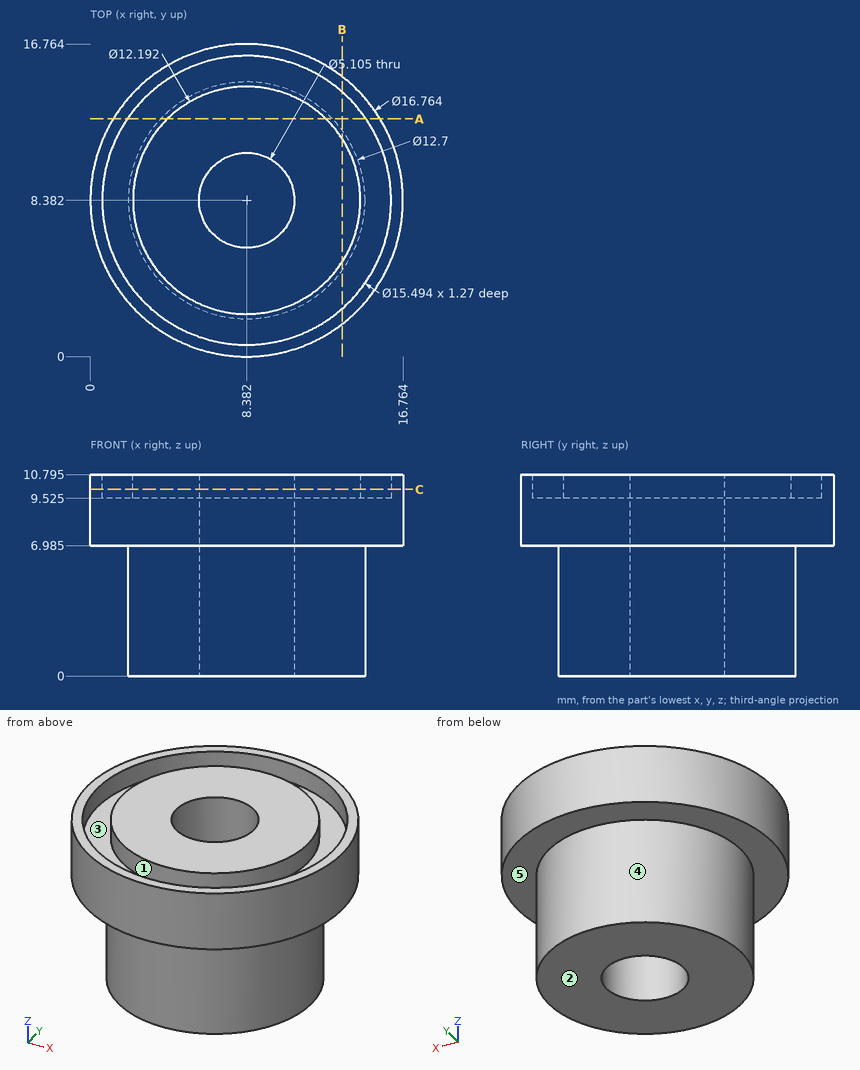
Part print with two shaded views. Sizes in mm from the minimum x, y, z corner. A direction names the side the tool comes from. Round coordinates to 2 decimals unless told otherwise and drop trailing zeros. Loops run counter-clockwise (first coordinate to the right, second up) from the corner with the lowest first, then second, coordinate; pieces in that order, holes last. Notation, with made-up numbers: M -15.75,28 L 7.25,28 A17 cw 7.25,38 Z; hole C 12,46 d1. An arc over 180 degrees is marked long. Return JSON: item names as keys, results as strings. Group by question number.
(1) Saw through at C-C, the plane z = 10. List the corners of the cut face in (x, y) (1 decimal).
(2) Drop flat-ended pins along their axis: P1, Ø3, axis at x = 10.5, y = 10, coming from the -Z side; P2, Ø3, axis at y = 3.5, z = 8.5, coming from the -X side; P3, Ø3, axis at y = 6, z = 4.5, coming from the +X side; P4, Ø6, axis at y = 4, z = 8, coming from the -X side (1 decimal). Give the stop position or say it passes through.
(3) Wall check: probe 1 along Y at (x, z) = (8.5, 10.25); probe 2 along Z at (x, y) = (3.75, 4) (1 decimal); probe 3 along Y at (x, z) = (8.25, 1.5). Give the ranges that are in metal, low to high. Write a range as [from, to].
(4) Mould opens along Y. For the marked faces 3, 4 and 5 say: +Y half, -Y half, draft (parallel to the pull), parting line (faces both ways), or undercut.
(5) Saw through at B-B, the plane x = 13.5. List the corners of the cut face in (y, z) (1 decimal).
(6) Saw through at A-A, the plane y = 12.75. List the corners of the cut face in (x, z) (1 decimal).
(7) Tool access for the marked faces 1 and 2: list every direction of +Z, -Z, +X, -X, +Y, -Y with a clear straight run to the whole face (end or side of a thin tool).
Answer list:
{
 "1": {"outline": "C 8.4,8.4 d16.8; C 8.4,8.4 d12.2; hole C 8.4,8.4 d15.5; hole C 8.4,8.4 d5.1"},
 "2": {"P1": "z = 0", "P2": "x = 0.71", "P3": "x = 14.67", "P4": "x = 0.1"},
 "3": {"probe 1": "[0, 0.64], [2.29, 5.83], [10.93, 14.48], [16.13, 16.76]", "probe 2": "[7, 9.5]", "probe 3": "[2.03, 5.83], [10.93, 14.73]"},
 "4": {"face 3": "undercut", "face 4": "parting line", "face 5": "draft"},
 "5": {"outline": "M 1.7,7 L 4.6,7 L 4.6,0 L 12.1,0 L 12.1,7 L 15,7 L 15,10.8 L 14.2,10.8 L 14.2,9.5 L 11.7,9.5 L 11.7,10.8 L 5.1,10.8 L 5.1,9.5 L 2.6,9.5 L 2.6,10.8 L 1.7,10.8 Z"},
 "6": {"outline": "M 1.2,7 L 3.8,7 L 3.8,0 L 13,0 L 13,7 L 15.5,7 L 15.5,10.8 L 14.8,10.8 L 14.8,9.5 L 12.6,9.5 L 12.6,10.8 L 4.1,10.8 L 4.1,9.5 L 2,9.5 L 2,10.8 L 1.2,10.8 Z"},
 "7": {"face 1": "+Z", "face 2": "-Z, +X, -X, +Y, -Y"}
}
